from build123d import *

# Parameters (mm, degrees)
BOSS_EXTRU_1_DEPTH      = 4
ENL_V_MAT_EXTRU_1_DEPTH = 2
CONG_4_R                = 7
CONG_3_R                = 0.9
CONG_5_R                = 1.5


with BuildPart() as part:
    # Esquisse1 → Boss.-Extru.1 (new, symmetric)
    with BuildSketch(Plane.XY):
        with BuildLine():
            Line((0, 0), (0, 9))
            Line((0, 9), (1, 9))
            Line((1, 9), (1, 0.09638948))
            Line((1, 0.09638948), (10.121873618, 0.09638948))
            ThreePointArc((10.121873618, 0.09638948), (32.996323667, 35.335168912), (70.121873618, 55))
            Line((70.121873618, 55), (70.121873618, 68.436194763))
            Line((70.121873618, 68.436194763), (60.432430442, 68.436194763))
            ThreePointArc((60.432430442, 68.436194763), (52.298183077, 58.663045958), (40.121873618, 55))
            Line((40.121873618, 55), (19.293191489, 55))
            Line((19.293191489, 55), (10.121873618, 55))
            Line((10.121873618, 55), (-4, 55))
            Line((-4, 55), (-4, 40))
            Line((-4, 40), (0, 40))
            Line((0, 40), (0, 49))
            Line((0, 49), (1, 49))
            Line((1, 49), (1, 15))
            Line((1, 15), (-4, 15))
            Line((-4, 15), (-4, 0))
            Line((-4, 0), (0, 0))
        make_face()
    extrude(amount=BOSS_EXTRU_1_DEPTH, both=True)

    # Esquisse4 → Enlèv. mat.-Extru.1 (cut)
    with BuildSketch(Plane.XY.offset(4)):
        Polygon((0, 40), (-4, 40), (-4, 55), (1, 55), (1, 40), align=None)
        Polygon((0, 0), (-4, 0), (-4, 15), (1, 15), (1, 0), align=None)
    extrude(amount=-ENL_V_MAT_EXTRU_1_DEPTH, mode=Mode.SUBTRACT)

    # Congé4
    # the kernel refuses this fillet: 7 mm, written as the material it takes off along each edge
    with BuildSketch(Plane(origin=(70.121873618, 68.436194763, -21.5), x_dir=(-1, 0, 0), z_dir=(0, 0, 1))) as cong_4_piece_1:
        with BuildLine():
            CenterArc((CONG_4_R, CONG_4_R), CONG_4_R, 180, 90)
            Line((0, CONG_4_R), (0, 0))
            Line((0, 0), (CONG_4_R, 0))
        make_face()
    extrude(amount=43, mode=Mode.SUBTRACT)
    with BuildSketch(Plane(origin=(60.432430442, 68.436194763, -14.492760312), x_dir=(-0.46608321311989886, -0.8847408877450115, 0), z_dir=(0, 0, 1))) as cong_4_piece_2:
        with BuildLine():
            CenterArc((4.236986438, 6.975932121), CONG_4_R, 207.780348291, 57.467043301)
            Line((-1.956199776, 3.713349629), (0, 0))
            ThreePointArc((0, 0), (1.828505702, 0.075879566), (3.657011403, 0))
        make_face()
    extrude(amount=28.985520624, mode=Mode.SUBTRACT)

    # Congé3
    # the kernel refuses this fillet: 0.9 mm, written as the material it adds along each edge
    with BuildSketch(Plane(origin=(1, 9, -4), x_dir=(-1, 0, 0), z_dir=(0, 0, 1)), Plane(origin=(0, 9, -4), x_dir=(0, -1, 0), z_dir=(0, 0, 1)), Plane(origin=(1, 15, -4), x_dir=(0, 1, 0), z_dir=(0, 0, 1))) as cong_3_piece_1:
        with BuildLine():
            CenterArc((CONG_3_R, CONG_3_R), CONG_3_R, 180, 90)
            Line((0, CONG_3_R), (0, 0))
            Line((0, 0), (CONG_3_R, 0))
        make_face()
    extrude(amount=6)
    with BuildSketch(Plane(origin=(1, 49, -4), x_dir=(0, -1, 0), z_dir=(0, 0, 1)), Plane(origin=(0, 49, -4), x_dir=(1, 0, 0), z_dir=(0, 0, 1))) as cong_3_piece_2:
        with BuildLine():
            CenterArc((CONG_3_R, -CONG_3_R), CONG_3_R, 90, 90)
            Line((0, -CONG_3_R), (0, 0))
            Line((0, 0), (CONG_3_R, 0))
        make_face()
    extrude(amount=6)
    # the kernel refuses this fillet: 0.9 mm, written as the material it takes off along each edge
    with BuildSketch(Plane(origin=(1, 0.09638948, -6.25), x_dir=(0, 1, 0), z_dir=(0, 0, 1))) as cong_3_2_piece_1:
        with BuildLine():
            CenterArc((CONG_3_R, -CONG_3_R), CONG_3_R, 90, 90)
            Line((0, -CONG_3_R), (0, 0))
            Line((0, 0), (CONG_3_R, 0))
        make_face()
    extrude(amount=12.5, mode=Mode.SUBTRACT)
    with BuildSketch(Plane(origin=(0, 0, 4.25), x_dir=(0, 1, 0), z_dir=(0, 0, -1)), Plane(origin=(-4, 0, 4.25), x_dir=(1, 0, 0), z_dir=(0, 0, -1))) as cong_3_2_piece_2:
        with BuildLine():
            CenterArc((CONG_3_R, -CONG_3_R), CONG_3_R, 90, 90)
            Line((0, -CONG_3_R), (0, 0))
            Line((0, 0), (CONG_3_R, 0))
        make_face()
    extrude(amount=10.5, mode=Mode.SUBTRACT)
    with BuildSketch(Plane(origin=(0, 40, -6.25), x_dir=(0, 1, 0), z_dir=(0, 0, 1)), Plane(origin=(-4, 40, -6.25), x_dir=(1, 0, 0), z_dir=(0, 0, 1))) as cong_3_2_piece_3:
        with BuildLine():
            CenterArc((CONG_3_R, CONG_3_R), CONG_3_R, 180, 90)
            Line((0, CONG_3_R), (0, 0))
            Line((0, 0), (CONG_3_R, 0))
        make_face()
    extrude(amount=10.5, mode=Mode.SUBTRACT)
    with BuildSketch(Plane(origin=(70.121873618, 55, -5.770556853), x_dir=(-0.9719612569458899, -0.2351410534044747, 0), z_dir=(0, 0, 1))) as cong_3_2_piece_4:
        with BuildLine():
            CenterArc((0.70823289, -0.899992014), CONG_3_R, 90.241370438, 76.15869203)
            Line((-0.166532241, -0.688365066), (0, 0))
            ThreePointArc((0, 0), (0.352220732, -0.000741903), (0.704441463, 0))
        make_face()
    extrude(amount=11.541113707, mode=Mode.SUBTRACT)
    with BuildSketch(Plane(origin=(10.121873618, 0.09638948, -5.615046517), x_dir=(-1, 0, 0), z_dir=(0, 0, 1))) as cong_3_2_piece_5:
        with BuildLine():
            CenterArc((0.646018607, -0.9), CONG_3_R, 90, 71.121872084)
            ThreePointArc((-0.205569441, -0.608799388), (-0.102199862, -0.304597179), (0, 0))
            Line((0, 0), (0.646018607, 0))
        make_face()
    extrude(amount=11.230093034, mode=Mode.SUBTRACT)

    # Congé5
    cong_5_edges = [part.edges().sort_by_distance(p)[0] for p in [
        (50.731308414, 57.717480203, -4),
        (60.938289065, 67.383858728, -4),
        (50.731308414, 57.717480203, 4),
        (60.938289065, 67.383858728, 4),
        (18.060936809, 55, -4),
        (20.560936809, 55, 4),
        (-4, 15, -1),
        (-4, 55, -1),
    ]]
    fillet(cong_5_edges, radius=CONG_5_R)


solid = part.part
Input: part model. Units: mm. Frame: model coordinates. A direction names the side the tool comes from. Coordinates: 2 decimals unless noted, no trailing zeros. Loops run counter-clockwise (first coordinate to the right, second up) from the corner with the lowest first, then second, coordinate; pieces in that order, holes last. Notation, with made-up numbers: (31.5, 44) -> (51.5, 44) arc R22 cw to (51.5, 71) -> close; hole circle Ø9 at (30, -36.75). An arc over 180 degrees is marked (long way). Write each question's results on one line, items separated by ' | '. Start each with the question number.
Q1. Pull-direction query (X, two-part tool) for faces 4 (the cylindrical face through (50.867, 57.792, 0.035)), 5 (the flat face through (0, 44, -1)), 6 (the flat face through (23, 39, 4)); classes: released by +X, released by -X, zero draft, split by the parting line, or undercut.
Q2. Section B-B, the plane y = 43. Return the cut outline in (x, z).
Q3. Ray query, line 1 (X direction, y = 42, z = -1); line 2 (Y direction, x = 26, z = 3); line 3 (X direction, y = 27, z = 1.75). Return the intervals inside material, ascending. Write a range as from..to.
Q4. Pin query (flat end, axial travel): pin 1 (4 mm diameter, centred on x = -2, y = 8.5, fed in from +Z); pin 2 (2 mm diameter, centred on y = 11.5, z = -1, fed in from +X); pin 3 (4 mm diameter, centred on x = 17, z = 1, fed in from +Y). Return the tip coordinate at first contact, or that it passes through.
Q5. Section D-D, the plane y = 51. Return the cut outline in (x, z), plus the area to 3 significant figures.
Q6. Section C-C, the plane x = 29.5. Return the cut outline in (y, z), plus the area to 3 significant figures.
Q7. Reachability of faces 1 (the flat face through (-2, 8, 2)), 2 (the flat face through (19, 55, 0)), 3 (the flat face through (0, 4, -1)) from +Z, -Z, +X, -X, +Y, -Y: full face, straight path, thin tool, end or side. Return the list, or none.
Found:
1) face 4: released by -X | face 5: undercut | face 6: zero draft
2) outline: (-4, -4) -> (0, -4) -> (0, 2) -> (-4, 2) -> close; (1, -4) -> (42.73, -4) -> (42.73, 4) -> (1, 4) -> close
3) line 1: -4..0, 1..41.28 | line 2: 28.11..54.91 | line 3: 1..25.06
4) pin 1: z = 2 | pin 2: x = 15.4 | pin 3: y = 55
5) outline: (-4, -4) -> (57.69, -4) -> (57.69, 4) -> (1, 4) -> (1, 2) -> (-4, 2) -> close | area: 484 mm2
6) outline: (31.94, -4) -> (53.5, -4) arc R1.5 ccw to (55, -2.5) -> (55, 2.5) arc R1.5 ccw to (53.5, 4) -> (31.94, 4) -> close | area: 183 mm2
7) face 1: +Z, -X, +Y, -Y | face 2: +Z, -Z, -X, +Y | face 3: +Z, -Z, -Y
